Part model, mm, in its own coordinate system. A direction names the side the tool comes from. Coordinates: 2 decimals unless noted, no trailing zeros. Loops run counter-clockwise (first coordinate to the right, second up) from the corner with the lowest first, then second, coordinate; pieces in that order, holes last. Notation, with made-up numbers: (2, -34.5) - (15, -34.5) arc R25 ccw to (15, -1.5) - close; hole circle Ø4 at (7, -7.5). An arc over 180 degrees is marked (long way). Use a Markdown table: item, result. Add a question column.
1. 3-axis set-ups, long thin cutter, end or side, ignore diameter. For faces 1 (the flat face through (-2.158, 9, 2)), 2 (the flat face through (-1.908, 4, 3)), 3 (the flat face through (1, 1, 3.77)), 4 (the flat face through (0, 3, -59)): which of +Z, -Z, +X, -X, +Y, -Y reach the whole face in a straight line?
2. Band-saw the part on A-A, the plane x = 10.75. Give the cut face in (y, z).
3. Drop flat-ended pins along their axis: pin 1 (1.2 mm diameter, centred on y = 8, z = 2, fed in from +X); pin 2 (0.9 mm diameter, centred on x = 0, z = -76.5, fed in from +Y); pin 3 (4.5 mm diameter, centred on y = 1, z = -63, fed in from -X); pin 4 (2.5 mm diameter, centred on x = 0, y = 2, fed in from -Z). Give the stop position or say it passes through.
4. Band-saw the part on B-B, the plane y = -2.5. Give the cut face in (x, z), plus the area to 3 significant figures.
5. Pull direction X, two halves, no side cores. Call faces 5 (the flat face through (-1.067, 1, -59)), 6 (the flat face through (-1.584, 1, -59)), 7 (the flat face through (0, -6.19, 4)): pulls with the +X half, pulls with the -X half, needs draft (parallel to the pull), parting line crosses it, or undercut.
6. Wall check: probe 1 along Y at (x, z) = (0, -28.5); probe 2 along Z at (x, y) = (0.5, 0.75); probe 3 along X at (y, z) = (2, -60). Give the ranges that are in metal, low to high. Write a range as [from, to].
7. Band-saw the part on C-C, the plane z = -75.5. Give the cut face in (x, y), plus the area to 3 significant figures.
from build123d import *

# Parameters (mm, degrees)
F1_DEPTH = 5
F2_R     = 0.5
F3_W     = 4.5
F3_H     = 2.5
F4_DEPTH = 25
F5_W     = 4.5
F5_H     = 2.5
F6_DEPTH = 25
F7_W     = 4
F7_H     = 4
F7_W_2   = 3
F7_H_2   = 3
F8_DEPTH = 120


with BuildPart() as f1:
    # F0 (on Top) → F1 (new body)
    with BuildSketch(Plane.XY):
        Polygon((-2.157534, 3.810042), (-12.157534, 3.810042), (-12.157534, -1.189958), (-2.157534, -1.189958), (-2.157534, -6.189958), (2.842466, -6.189958), (2.842466, -1.189958), (12.842466, -1.189958), (12.842466, 3.810042), (2.842466, 3.810042), (2.842466, 13.810042), (-2.157534, 13.810042), align=None)
    extrude(amount=F1_DEPTH)

    # F2
    f2_edges = [f1.edges().sort_by_distance(p)[0] for p in [
        (-2.157534, 8.810042, 5),
        (-7.157534, 3.810042, 5),
        (-12.157534, 1.310042, 5),
        (-7.157534, -1.189958, 5),
        (-2.157534, -3.689958, 5),
        (0.342466, -6.189958, 5),
        (2.842466, -3.689958, 5),
        (7.842466, -1.189958, 5),
        (12.842466, 1.310042, 5),
        (7.842466, 3.810042, 5),
        (2.842466, 8.810042, 5),
        (0.342466, 13.810042, 5),
        (-2.157534, 8.810042, 0),
        (-7.157534, 3.810042, 0),
        (-12.157534, 1.310042, 0),
        (-7.157534, -1.189958, 0),
        (-2.157534, -3.689958, 0),
        (0.342466, -6.189958, 0),
        (2.842466, -3.689958, 0),
        (7.842466, -1.189958, 0),
        (12.842466, 1.310042, 0),
        (7.842466, 3.810042, 0),
        (2.842466, 8.810042, 0),
        (0.342466, 13.810042, 0),
    ]]
    fillet(f2_edges, radius=F2_R)

    # F3 (on Right) → F4 (cut, symmetric)
    with BuildSketch(Plane.YZ):
        with Locations((1.310042, 2.520103)):
            Rectangle(F3_W, F3_H)
    extrude(amount=F4_DEPTH, both=True, mode=Mode.SUBTRACT)

    # F5 (on Front) → F6 (cut, symmetric)
    with BuildSketch(Plane.XZ):
        with Locations((0.342466, 2.519919)):
            Rectangle(F5_W, F5_H)
    extrude(amount=F6_DEPTH, both=True, mode=Mode.SUBTRACT)

    # F7 (on Top) → F8 (join)
    with BuildSketch(Plane.XY):
        with Locations((0.416273, 1.462451)):
            Rectangle(F7_W, F7_H)
        with Locations((0.432896, 1.5)):
            Rectangle(F7_W_2, F7_H_2, mode=Mode.SUBTRACT)
    extrude(amount=-F8_DEPTH)


solid = f1.part
Geometry check:
| question | item | result |
|---|---|---|
| 1 | face 1 | +Z, -Z, -X, +Y |
| 1 | face 2 | +Y, -Y |
| 1 | face 3 | +X, -X |
| 1 | face 4 | -Z |
| 2 | outline | (-1.19, 0.5) arc R0.5 ccw to (-0.69, 0) - (3.31, 0) arc R0.5 ccw to (3.81, 0.5) - (3.81, 4.5) arc R0.5 ccw to (3.31, 5) - (-0.69, 5) arc R0.5 ccw to (-1.19, 4.5) - close; hole (-0.94, 1.27) - (3.56, 1.27) - (3.56, 3.77) - (-0.94, 3.77) - close |
| 3 | pin 1 | stops at x = 2.84 |
| 3 | pin 2 | stops at y = 3.46 |
| 3 | pin 3 | stops at x = -1.58 |
| 3 | pin 4 | stops at z = -120 |
| 4 | outline | (-2.16, 0.5) arc R0.5 ccw to (-1.66, 0) - (2.34, 0) arc R0.5 ccw to (2.84, 0.5) - (2.84, 4.5) arc R0.5 ccw to (2.34, 5) - (-1.66, 5) arc R0.5 ccw to (-2.16, 4.5) - close; hole (-1.91, 1.27) - (2.59, 1.27) - (2.59, 3.77) - (-1.91, 3.77) - close |
| 4 | area | 13.5 mm^2 |
| 5 | face 5 | undercut |
| 5 | face 6 | pulls with the -X half |
| 5 | face 7 | needs draft |
| 6 | probe 1 | y = [-0.54, 0], [3, 3.46] |
| 6 | probe 2 | z = [0, 1.27], [3.77, 5] |
| 6 | probe 3 | x = [-1.58, -1.07], [1.93, 2.42] |
| 7 | outline | (-1.58, -0.54) - (2.42, -0.54) - (2.42, 3.46) - (-1.58, 3.46) - close; hole (-1.07, 0) - (1.93, 0) - (1.93, 3) - (-1.07, 3) - close |
| 7 | area | 7.00 mm^2 |
